Read the model definition and answer for the solid it produces. Units are mm, in the model's axes. Face numbers are marked on the shaded views. A direction names the side the tool comes from. Coordinates: 2 decimals unless noted, no trailing zeros. Loops run counter-clockwise (first coordinate to the right, second up) from the corner with the lowest first, then second, coordinate; pieces in that order, holes last.
from build123d import *

# Parameters (mm, degrees)
SKETCH_1_R          = 1.95
EXTRUDE_1_DEPTH     = 12
SKETCH_4_W          = 2
SKETCH_4_H          = 9
EXTRUDE_2_DEPTH     = 1.95
EXTRUDE_4_DEPTH     = 8.8
SKETCH_9_R          = 2
CUT_EXTRUDE_2_DEPTH = 17
SKETCH_13_R         = 2.75
CUT_EXTRUDE_6_DEPTH = 1
CUT_EXTRUDE_7_DEPTH = 13.389713


with BuildPart() as part:
    # 스케치1 → 보스-돌출1 (new body)
    with BuildSketch(Plane.XY):
        Circle(SKETCH_1_R)
    extrude(amount=EXTRUDE_1_DEPTH)

    # 스케치4 → 보스-돌출2 (add)
    with BuildSketch(Plane(origin=(0, 0, 0), x_dir=(0, 0, -1), z_dir=(1, 0, 0))):
        with Locations((-1, -2.55)):
            Rectangle(SKETCH_4_W, SKETCH_4_H)
    extrude(amount=EXTRUDE_2_DEPTH)

    # 스케치8 → 보스-돌출4 (add)
    with BuildSketch(Plane.XY.offset(2)):
        with BuildLine():
            ThreePointArc((1.95, -1.643168), (1.075273, -2.312204), (0, -2.55))
            Line((0, -2.55), (0, -7.05))
            Line((0, -7.05), (1.95, -7.05))
            Line((1.95, -7.05), (1.95, -1.643168))
        make_face()
    extrude(amount=EXTRUDE_4_DEPTH)

    # 스케치9 → 컷-돌출2 (cut)
    with BuildSketch(Plane.ZY):
        with Locations((5.5, -7.55)):
            Circle(SKETCH_9_R)
    extrude(amount=-CUT_EXTRUDE_2_DEPTH, mode=Mode.SUBTRACT)

    # 스케치13 → 컷-돌출6 (cut)
    with BuildSketch(Plane.ZY):
        with Locations((5.505014, -7.55)):
            Circle(SKETCH_13_R)
    extrude(amount=-CUT_EXTRUDE_6_DEPTH, mode=Mode.SUBTRACT)

    # 스케치12 → 컷-돌출7 (cut, through all)
    with BuildSketch(Plane.XY.offset(2)):
        with BuildLine():
            Line((1.95, 0), (1.95, 1.95))
            Line((1.95, 1.95), (0, 1.95))
            ThreePointArc((0, 1.95), (1.378858, 1.378858), (1.95, 0))
        make_face()
    extrude(amount=-CUT_EXTRUDE_7_DEPTH, mode=Mode.SUBTRACT)


solid = part.part
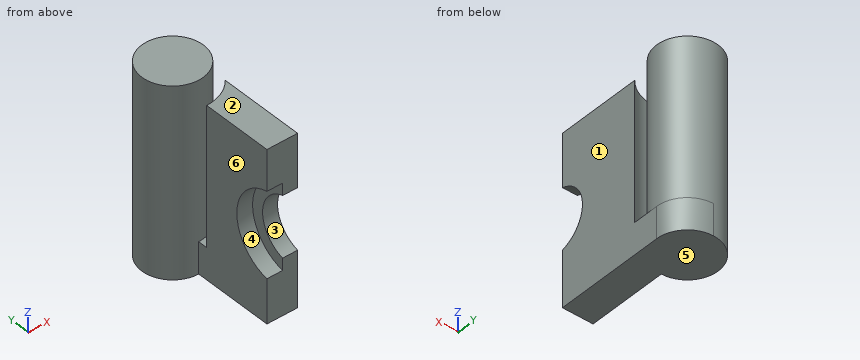
Q1. A cutting plane is placed at B-B (x = 1.55). Give the vertices of the cut face in (y, z), then the cut area to 3 significant figures.
Findings below:
outline: (-7.05, 0) - (1.18, 0) - (1.18, 12) - (-1.18, 12) - (-1.18, 2) - (-2.02, 2) - (-2.02, 10.8) - (-7.05, 10.8) - (-7.05, 7.44) arc R2 cw to (-7.05, 3.56) - close
area: 80.0 mm2
Q2. A cutting plane is placed at D-D (z = 6). Give the vertices of the cut face in (x, y), then the cut area to 3 significant figures.
Findings below:
outline: circle Ø3.9 at (0, 0); (0, -4.84) - (1, -4.84) - (1, -5.61) - (1.95, -5.61) - (1.95, -1.64) arc R2.55 cw to (0, -2.55) - close
area: 17.7 mm2
Q3. Which of the six approach directions +Z, -Z, +X, -X, +Y, -Y give full straight-line access (tool end or side, diameter ignored) to the marked faces 4, 5 and 6?
Findings below:
face 4: -X, -Y
face 5: -Z, +X, -X, +Y, -Y
face 6: +Z, -Z, -X, -Y
Q4. Determine the mould class of the marked faces 1, 2 and 3 for opening direction Z: +Z half, -Z half, draft (parallel to the pull), parting line (faces both ways), or undercut.
Findings below:
face 1: draft
face 2: +Z half
face 3: undercut
Q5. Flat-ended cylindrical pins translate along their axes: pin 1 Ø2.5 at (y, z) = (-5.5, 6) entering from -X; pin 2 Ø1 at (y, z) = (1, 4) entering from +X; pin 3 Ø2 at (x, y) = (1.5, -5.5) entering from +Z. Find the tip coordinate at first contact, or state that the pin passes through.
Findings below:
pin 1: stops at x = 0
pin 2: stops at x = 1.88
pin 3: stops at z = 10.8
Q6. A cutting plane is placed at C-C (y = -0.75). Give the vertices of the cut face in (x, z).
Findings below:
outline: (-1.8, 0) - (1.95, 0) - (1.95, 2) - (1.8, 2) - (1.8, 12) - (-1.8, 12) - close
Q7. Straight lines are drawn through the part: probe 1 along Y at (x, z) = (0.05, 11.25); probe 2 along X at (y, z) = (-3.75, 10.25); probe 3 along Y at (x, z) = (1.2, 10.75). For each, find the intervals that lie inside material, in ascending order.
Findings below:
probe 1: y = -1.95 to 1.95
probe 2: x = 0 to 1.95
probe 3: y = -7.05 to -2.25, -1.54 to 1.54
Q8. A cutting plane is placed at A-A (z = 9.25). Give the vertices of the cut face in (x, y).
Findings below:
outline: circle Ø3.9 at (0, 0); (0, -7.05) - (1.95, -7.05) - (1.95, -1.64) arc R2.55 cw to (0, -2.55) - close
